For this review, take the finished solid that the model builds, in its own axes (mm). Give positions to 0.01 mm unless a question says otherwise; leave off trailing zeros. Loops run counter-clockwise (first coordinate to the right, second up) from the corner with the lowest first, then second, coordinate; pieces in that order, holes last.
Autodesk Inventor part; units mm, degrees
ref_plane "YZ Plane" through (0, 0, 0) normal (1, 0, 0) x (0, 1, 0)
ref_plane "XZ Plane" through (0, 0, 0) normal (0, 1, 0) x (-1, 0, 0)
ref_plane "XY Plane" through (0, 0, 0) normal (0, 0, 1) x (1, 0, 0)
sketch "Szkic1" plane through (0, 0, 0) normal (0, 0, 1) x (1, 0, 0)
  line L0 (-47.736, 26.7667) -> (-47.736, 6.7667)
  line L1 (-47.736, 26.7667) -> (52.264, 26.7667)
  line L2 (52.264, 26.7667) -> (52.264, 6.7667)
  line L3 (52.264, 6.7667) -> (32.264, 6.7667)
  line L4 (32.264, 6.7667) -> (32.264, -48.2333)
  line L5 (32.264, -48.2333) -> (-27.736, -48.2333)
  line L6 (-27.736, -48.2333) -> (-27.736, 6.7667)
  line L7 (-27.736, 6.7667) -> (-47.736, 6.7667)
  circle A0 centre (2.264, -27.7333) radius 19
  arc A1 (-11.0025, -7.7333) -> (-11.0025, -47.7333) centre (2.264, -27.7333) ccw
  line L8 (-11.0025, -47.7333) -> (15.5305, -47.7333)
  arc A2 (15.5305, -47.7333) -> (15.5305, -7.7333) centre (2.264, -27.7333) ccw
  line L9 (15.5305, -7.7333) -> (-11.0025, -7.7333)
  circle A3 centre (2.264, -27.7333) radius 15
  circle A4 centre (-37.736, 16.7667) radius 2
  circle A5 centre (2.264, 16.7667) radius 2
  circle A6 centre (42.264, 16.7667) radius 2
  arc A7 (-23.5765, -30.609) -> (-13.7282, -48.2333) centre (2.264, -27.7333) ccw
  arc A8 (18.2561, -48.2333) -> (28.1044, -30.609) centre (2.264, -27.7333) ccw
  line L10 (-27.736, 6.7667) -> (-23.5765, -30.609)
  line L11 (32.264, 6.7667) -> (28.1044, -30.609)
  line L12 (-7.736, 26.7667) -> (-7.736, 66.7667)
  line L13 (-7.736, 66.7667) -> (12.264, 66.7667)
  line L14 (12.264, 66.7667) -> (12.264, 26.7667)
  circle A9 centre (2.264, 56.7667) radius 2
  line L15 (-27.736, 6.7667) -> (32.264, 6.7667)
  point P0 (0, 0)
  point P1 (-16.736, -27.7333)
  point P2 (-11.1711, -41.1683)
  point P3 (15.699, -14.2982)
  point P4 (15.699, -41.1683)
  point P5 (-11.1711, -14.2982)
  point P6 (21.264, -27.7333)
  dimension "d0" = 20
  dimension "d1" = 100
  dimension "d2" = 20
  dimension "d3" = 60
  dimension "d4" = 20
  dimension "d5" = 55
  dimension "d8" = 38
  dimension "d13" = 34.5
  dimension "d14" = 30
  dimension "d15" = 30
  dimension "d24" = 4
  dimension "d25" = 4
  dimension "d26" = 4
  dimension "d29" = 10
  dimension "d30" = 10
  dimension "d31" = 10
  dimension "d32" = 10
  dimension "d33" = 10
  dimension "d34" = 50
  dimension "d42" = 2
  dimension "d47" = 40
  dimension "d48" = 20
  dimension "d49" = 40
  dimension "d50" = 10
  dimension "d51" = 10
  dimension "d52" = 4
extrude "Wyciągnięcie proste1" add sketch "Szkic1" along normal blind 20 contours L1 L2 L3 L15 L7 L0 | L12 L13 L14 L1 | L10 A7 L5 L6 | L15 L11 A8 L5 A7 L10 | L4 L5 A8 L11 | A0 | L9 A2 L8 A1 | A3 | A4 | A5 | A6 | A9
extrude "Wyciągnięcie proste2" cut sketch "Szkic1" along normal through all contours A3 | A4 | A5 | A6 | A9
hole "Otwór1" at (2.264, -27.7333, 0) at (21.264, -27.7333, 0) at (-11.1711, -41.1683, 0) at (15.699, -41.1683, 0) at (15.699, -14.2982, 0) at (-11.1711, -14.2982, 0) at (-16.736, -27.7333, 0) direction (0, 0, 1) diameter 5 end through all
extrude "Wyciągnięcie proste3" cut sketch "Szkic1" along normal through all contours L10 A7 L5 L6 | L4 L5 A8 L11
extrude "Wyciągnięcie proste4" cut sketch "Szkic1" along normal through all contours L1 L2 L3 L15 L7 L0 | L12 L13 L14 L1
fillet "Zaokrąglenie3" radius 4 2 edges at (32.264, 6.7667, 10) (-27.736, 6.7667, 10)
fillet "Zaokrąglenie4" radius 8 2 edges at (-13.7282, -48.2333, 10) (18.2561, -48.2333, 10)
equation "\"d2\" = -0.5 * d3 + 0.5 * d1"
equation "\"d34\" = 0.5 * d1"
properties part number "3DP_ABS_Heatbed_Frame_Ball_Screw_Nut_Mounting_Bracket_Filler"
Q1. Mouldability with a two-part tool opening along Y and no side actions: class faces 1 (the cylindrical face through (-10.21, -38.86, 10.14)), 2 (the flat face through (2, -8, 0)), 3 (the flat face through (29.963, -13.912, 9.86)) as +Y half, -Y half, draft (parallel to the pull), parting line (faces both ways), or undercut.
Answers:
face 1: undercut
face 2: draft
face 3: -Y half
Q2. For probe 1 along Y at (x, z) = (2, 4.75); probe 2 along X at (y, z) = (-40.5, 2.75); probe 3 along X at (y, z) = (-28.5, 8.5), list the stretches that pass through material, from the lowest coordinate up.
Answers:
probe 1: y = -48.23 to -42.73, -12.74 to 6.77
probe 2: x = -20.39 to -13.58, -8.76 to -5.61, 10.14 to 13.29, 18.11 to 24.91
probe 3: x = -23.81 to -19.12, -14.36 to -12.72, 17.24 to 18.88, 23.64 to 28.34
Q3. For pin 1 Ø1.5 at (y, z) = (-26.5, 4) entering from -X; pin 2 Ø1.5 at (y, z) = (-11.5, 7.5) entering from -X; pin 3 Ø2 at (y, z) = (-6.5, 4) entering from -X, all flat-tipped, find the tip position at first contact; note any pin that passes through.
Answers:
pin 1: stops at x = -24.12
pin 2: stops at x = -25.79
pin 3: stops at x = -26.37
Q4. Consider section D-D on y = -40.5. Give the boundary of the cut face in (x, z), plus the area to 3 significant figures.
Answers:
outline: (-20.39, 0) - (-13.58, 0) - (-13.58, 20) - (-20.39, 20) - close; (-8.76, 0) - (-5.61, 0) - (-5.61, 20) - (-8.76, 20) - close; (10.14, 0) - (13.29, 0) - (13.29, 20) - (10.14, 20) - close; (18.11, 0) - (24.91, 0) - (24.91, 20) - (18.11, 20) - close
area: 398 mm2
Q5. Consider section C-C on z = 12.75. Give the boundary of the cut face in (x, y).
Answers:
outline: (-27.24, 2.32) - (-23.58, -30.61) arc R26 ccw to (-16.44, -45.79) arc R8 ccw to (-10.69, -48.23) - (15.22, -48.23) arc R8 ccw to (20.97, -45.79) arc R26 ccw to (28.1, -30.61) - (31.77, 2.32) arc R4 ccw to (27.79, 6.77) - (-23.27, 6.77) arc R4 ccw to start; hole circle Ø5 at (-16.74, -27.73); hole circle Ø5 at (-11.17, -41.17); hole circle Ø5 at (-11.17, -14.3); hole circle Ø30 at (2.26, -27.73); hole circle Ø5 at (15.7, -41.17); hole circle Ø5 at (15.7, -14.3); hole circle Ø5 at (21.26, -27.73)
Q6. Consider section B-B on y = -33.5. Give the boundary of the cut face in (x, z).
Answers:
outline: (-23.09, 0) - (-11.58, 0) - (-11.58, 20) - (-23.09, 20) - close; (16.11, 0) - (27.62, 0) - (27.62, 20) - (16.11, 20) - close
Q7. Consider section A-A on x = 3. Give the boundary of the cut face in (y, z), plus the area to 3 significant figures.
Answers:
outline: (-48.23, 0) - (-42.72, 0) - (-42.72, 20) - (-48.23, 20) - close; (-12.75, 0) - (6.77, 0) - (6.77, 20) - (-12.75, 20) - close
area: 501 mm2
